```python
from build123d import *

# Parameters (mm, degrees)
BOSS_EXTRU_1_DEPTH = 5
ESQUISSE2_W        = 5
ESQUISSE2_H        = 3
ESQUISSE2_H_2      = 7.0925
ESQUISSE2_W_2      = 3
ESQUISSE2_H_3      = 5
ESQUISSE2_W_3      = 2
ESQUISSE2_W_4      = 8.154681838
ESQUISSE2_W_5      = 10
CR_NEAUX_DEPTH     = 5
ESQUISSE3_R        = 0.5
PER_AGES_DEPTH     = 5


with BuildPart() as part:
    # Esquisse1 → Boss.-Extru.1 (new body)
    with BuildSketch(Plane.XY):
        Polygon((-40.2, 0), (-40.2, -19.685), (0, -19.685), (0, 0), (10, 0), (10, -32.401636706), (-115, -32.401636706), (-147.401636706, 0), (-112.246954868, 0), (-112.246954868, -17.5925), (-71.384202009, -17.5925), (-71.384202009, -24.685), (-52.2, -24.685), (-52.2, 0), align=None)
    extrude(amount=BOSS_EXTRU_1_DEPTH)

    # Esquisse2 → Créneaux - (cut)
    with BuildSketch(Plane(origin=(0, 0, 0), x_dir=(-1, 0, 0), z_dir=(0, 0, -1))):
        with Locations((4.65, -21.185)):
            Rectangle(ESQUISSE2_W, ESQUISSE2_H)
        with Locations((89.250434868, -21.13875)):
            Rectangle(ESQUISSE2_W, ESQUISSE2_H_2)
        with Locations((4.65, -30.901636706)):
            Rectangle(ESQUISSE2_W, ESQUISSE2_H)
        with Locations((-8.5, -2.5)):
            Rectangle(ESQUISSE2_W_2, ESQUISSE2_H_3)
        with Locations((-1, -2.5)):
            Rectangle(ESQUISSE2_W_3, ESQUISSE2_H_3)
        with Locations((41.2, -2.5)):
            Rectangle(ESQUISSE2_W_3, ESQUISSE2_H_3)
        with Locations((49.7, -2.5)):
            Rectangle(ESQUISSE2_W, ESQUISSE2_H_3)
        with Locations((114.746954868, -2.5)):
            Rectangle(ESQUISSE2_W, ESQUISSE2_H_3)
        with Locations((127.324295787, -2.5)):
            Rectangle(ESQUISSE2_W_4, ESQUISSE2_H_3)
        with Locations((142.401636706, -2.5)):
            Rectangle(ESQUISSE2_W_5, ESQUISSE2_H_3)
    extrude(amount=-CR_NEAUX_DEPTH, mode=Mode.SUBTRACT)

    # Esquisse3 → Perçages (cut)
    with BuildSketch(Plane(origin=(0, 0, 0), x_dir=(-1, 0, 0), z_dir=(0, 0, -1))):
        with Locations((-4.064, -14.986)):
            Circle(ESQUISSE3_R)
        with Locations((-4.064, -4.699)):
            Circle(ESQUISSE3_R)
        with Locations((44.264, -14.986)):
            Circle(ESQUISSE3_R)
        with Locations((44.264, -4.699)):
            Circle(ESQUISSE3_R)
    extrude(amount=-PER_AGES_DEPTH, mode=Mode.SUBTRACT)


solid = part.part
```
Source: CAD feature listing. Evaluate the final solid. Frame: model axes, mm. A direction names the side the tool comes from. Round coordinates to 2 decimals unless told otherwise and drop trailing zeros. Loops run counter-clockwise (first coordinate to the right, second up) from the corner with the lowest first, then second, coordinate; pieces in that order, holes last.
(1) Material intervals for probe 1 along X at (y, z) = (-3.5, 4.45); probe 2 along X at (y, z) = (-17, 3.3); probe 3 along X at (y, z) = (-24, 1.85), sorted ascending.
From the geometry:
probe 1: x = -137.4 to -131.4, -123.25 to -117.25, -47.2 to -42.2, 2 to 7
probe 2: x = -130.4 to -112.25, -52.2 to -40.2, 0 to 10
probe 3: x = -123.4 to -91.75, -86.75 to -71.38, -52.2 to 10
(2) Section query D-D (x = -88.5). Output: boundary loops of the cut face in (y, z) (3 decimals), and give its area (3 significant figures).
From the geometry:
outline: (-32.402, 0) - (-24.685, 0) - (-24.685, 5) - (-32.402, 5) - close
area: 38.6 mm2
(3) Section query A-A (y = -9). Output: boundary loops of the cut face in (x, z).
From the geometry:
outline: (-138.4, 0) - (-112.25, 0) - (-112.25, 5) - (-138.4, 5) - close; (-52.2, 0) - (-40.2, 0) - (-40.2, 5) - (-52.2, 5) - close; (0, 0) - (10, 0) - (10, 5) - (0, 5) - close
(4) Pull-direction query (X, two-part tool) for faces 5 (the flat face through (-127, -5, 2)), 6 (the flat face through (9, -5, 2)), 7 (the flat face through (7, -3, 2)); classes: +X half, -X half, draft (parallel to the pull), parting line (faces both ways), or undercut.
From the geometry:
face 5: undercut
face 6: draft
face 7: +X half
(5) Section query C-C (z = 3.3). Give the number of separate pieces and of enclosed holes in the cut face, and give its area (3 significant figures).
From the geometry:
separate pieces: 1
enclosed holes: 4
area: 2,360 mm2
(6) Access query for faces 1 (the flat face through (-47.2, -3, 2)), 2 (the flat face through (-140, -5, 2)), 3 (the flat face through (-5, -29.402, 2)), 4 (the flat face through (-60, -32.402, 2)). Directions: +Z, -Z, +X, -X, +Y, -Y. A direction counts if a zero-diameter tool reaches every point of the face in a straight line with its end or side. Return the directions, or none.
From the geometry:
face 1: +Z, -Z, +Y
face 2: +Z, -Z, -X, +Y
face 3: +Z, -Z, -Y
face 4: +Z, -Z, +X, -X, -Y
(7) Contact query for flat-ended pins moving along their axis: pin 1 Ø1.5 at (x, z) = (9, 1.5) entering from +Y; pin 2 Ø1.5 at (y, z) = (-2.5, 3.5) entering from +X; pin 3 Ø2 at (x, z) = (-125, 1) entering from -Y. Output: stop coordinate, or through.
From the geometry:
pin 1: stops at y = -5
pin 2: stops at x = 7
pin 3: stops at y = -23.4
(8) Section query B-B (x = -106.5). Output: boundary loops of the cut face in (y, z), and give its area (3 significant figures).
From the geometry:
outline: (-32.4, 0) - (-17.59, 0) - (-17.59, 5) - (-32.4, 5) - close
area: 74.0 mm2
